```python
from build123d import *

# Parameters (mm, degrees)
EXTRUDE_THIN1_DEPTH = 150.8125
FILLET1_R           = 1.016


with BuildPart() as part:
    # Sketch1 → Extrude-Thin1 (new body)
    with BuildSketch(Plane.XY):
        with BuildLine():
            ThreePointArc((0, 0), (-5.159375, -5.159375), (-10.31875, 0))
            Line((-10.31875, 0), (-10.31875, 4.365625))
            Line((-10.31875, 4.365625), (-12.7, 4.365625))
            Line((-12.7, 4.365625), (-12.7, 9.921875))
            Line((-12.7, 9.921875), (0, 9.921875))
            Line((0, 9.921875), (0, 8.905875))
            Line((0, 8.905875), (-11.684, 8.905875))
            Line((-11.684, 8.905875), (-11.684, 5.381625))
            Line((-11.684, 5.381625), (-9.30275, 5.381625))
            Line((-9.30275, 5.381625), (-9.30275, 0))
            ThreePointArc((-9.30275, 0), (-5.159375, -4.143375), (-1.016, 0))
            Line((-1.016, 0), (0, 0))
        make_face()
    extrude(amount=-EXTRUDE_THIN1_DEPTH)

    # Fillet1
    fillet1_edges = [part.edges().sort_by_distance(p)[0] for p in [
        (-9.30275, 5.381625, -75.40625),
        (-12.7, 4.365625, -75.40625),
        (-12.7, 9.921875, -75.40625),
    ]]
    fillet(fillet1_edges, radius=FILLET1_R)


solid = part.part
```
Check sheet for the modelled part. Datum: model origin and axes. Units: mm. A direction names the side the tool comes from. Give positions to 0.01 mm unless a question says otherwise; leave off trailing zeros. Order: outer loops, then holes, each group sorted by start corner. A loop starts at its lowest first (then second) coordinate and runs counter-clockwise, first axis right, second up. Notation, with made-up numbers: M -33,-4.5 L 23,-4.5 A37 cw 23,34.5 Z; hole C -24,77 d9. An arc over 180 degrees is marked long. Answer in a Markdown table with one row per item. Add a question column.
Q1. Sectioned sample at B-B, the plane x = -5.5. Record the boundary of the cut face in (y, z).
Q2. Gauge pin test, flat ends, axial feed: pin 1 Ø4 at (y, z) = (-2.5, -89) entering from +X; pin 2 Ø5 at (x, y) = (-5, -1.5) entering from +Z; pin 3 Ø1.1 at (y, z) = (7, -48.5) entering from +X. Record the tip position at first contact, or that the pin passes through.
Q3. Access from +Z, -Z, +X, -X, +Y, -Y to the whole of each face (thin tool, end or side, straight path). Record for faces 4 (the flat face through (-12.7, 7, -74)), 5 (the flat face through (-6, 8.906, -74)), 6 (the cylindrical face through (-5.25, -4.142, -74.351)), 7 (the flat face through (-6, 9.922, -74)), 8 (the flat face through (-10.319, 2, -74)).
Q4. Sectioned sample at A-A, the plane y = -2.25. Record the boundary of the cut face in (x, z).
Q5. Thickness scan on L1, parallel to X at y = -0.5, z = -16.5; L2, parallel to Y at x = -4.75, z = -5.5; L3, parallel to X at y = 7.25, z = -11. Record the ranges inside material, lowest first.
Q6. Sectioned sample at D-D, the plane y = 7.5. Record the boundary of the cut face in (x, z).
Q7. Release check for a two-part mould opening along Y. For faces 1 (the cylindrical face through (-5.05, -5.16, -74.35)), 2 (the flat face through (-10, 3, 0)), 3 (the flat face through (-9.303, 2, -74)) record: released by +Y, released by -Y, zero draft, split by the parting line, or undercut.
Q8. Sectioned sample at C-C, the plane z = -43.5. Record the boundary of the cut face in (x, y), and give its area (3 significant figures).
Verdict:
| question | item | result |
|---|---|---|
| 1 | outline | M -5.15,-150.81 L -4.13,-150.81 L -4.13,0 L -5.15,0 Z; M 8.91,-150.81 L 9.92,-150.81 L 9.92,0 L 8.91,0 Z |
| 2 | pin 1 | x = -0.02 |
| 2 | pin 2 | through |
| 2 | pin 3 | x = -11.68 |
| 3 | face 4 | +Z, -Z, -X, +Y, -Y |
| 3 | face 5 | +Z, -Z, +X |
| 3 | face 6 | +Z, -Z |
| 3 | face 7 | +Z, -Z, +X, -X, +Y |
| 3 | face 8 | +Z, -Z, -X, -Y |
| 4 | outline | M -9.8,-150.81 L -8.64,-150.81 L -8.64,0 L -9.8,0 Z; M -1.68,-150.81 L -0.52,-150.81 L -0.52,0 L -1.68,0 Z |
| 5 | L1 | -10.29 to -9.27, -1.05 to -0.02 |
| 5 | L2 | -5.14 to -4.12, 8.91 to 9.92 |
| 5 | L3 | -12.7 to -11.68 |
| 6 | outline | M -12.7,-150.81 L -11.68,-150.81 L -11.68,0 L -12.7,0 Z |
| 7 | face 1 | released by -Y |
| 7 | face 2 | zero draft |
| 7 | face 3 | undercut |
| 8 | outline | M -12.7,5.38 A1.02 ccw -11.68,4.37 L -10.32,4.37 L -10.32,0 A5.16 ccw 0,0 L -1.02,0 A4.14 cw -9.3,0 L -9.3,4.37 A1.02 ccw -10.32,5.38 L -11.68,5.38 L -11.68,8.91 L 0,8.91 L 0,9.92 L -11.68,9.92 A1.02 ccw -12.7,8.91 Z |
| 8 | area | 38.6 mm² |
